from build123d import *

# Parameters (mm, degrees)
SKETCH1_W           = 565.88
SKETCH1_H           = 129.88
BOSS_EXTRUDE1_DEPTH = 3.5
SKETCH2_R           = 20
BOSS_EXTRUDE2_DEPTH = 14


with BuildPart() as part:
    # Sketch1 → Boss-Extrude1 (new, symmetric)
    with BuildSketch(Plane.XY):
        Rectangle(SKETCH1_W, SKETCH1_H)
    extrude(amount=BOSS_EXTRUDE1_DEPTH, both=True)

    # Sketch2 → Boss-Extrude2 (add)
    with BuildSketch(Plane.XY.offset(3.5)):
        with Locations((-70, 0)):
            Circle(SKETCH2_R)
    extrude(amount=BOSS_EXTRUDE2_DEPTH)


solid = part.part
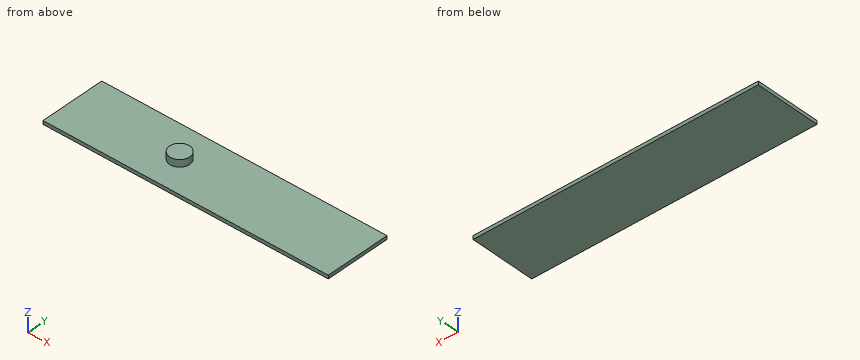
Can you work these out from the model? Positions are in its coordinate system, mm. Round coordinates to 2 decimals unless told otherwise and drop trailing zeros. Loops run counter-clockwise (first coordinate to the right, second up) from the corner with the lowest first, then second, coordinate; pieces in that order, holes last. Notation, with made-up numbers: (60.5, -30.5) - (111.5, -30.5) arc R12 cw to (111.5, -22.5) - close; hole circle Ø8 at (74.25, 26). An arc over 180 degrees is marked (long way). Answer in a Markdown table with one row per item. Add a question column.
Q1. I want a section at B-B on x = -70. List the corners of the cut face in (y, z) for me, and give its area (3 significant figures).
Q2. I want a section at D-D on y = -30. List the corners of the cut face in (x, z) for me, and give its area (3 significant figures).
Q3. I want a section at A-A on y = 0. List the corners of the cut face in (x, z) for me, and give its area (3 significant figures).
Q4. I need wall thicknesses on L1, parallel to Z at x = 21, y = -26.5; L2, parallel to X at y = 11, z = 7; L3, parallel to X at y = -13, z = 11.75. Which ranges of each line are inside material? Lowest first, please.
Q5. For pin 1 Ø10 at (x, y) = (153.5, -41) entering from +Z; pin 2 Ø6 at (y, z) = (-45.5, 4.5) entering from +X; pin 3 Ø1.5 at (y, z) = (42, 5) entering from -X, each with a flat end and sliding along its axis, tell me the tip position at first contact or that it passes through.
Q6. I want a section at C-C on z = 10.5. List the corners of the cut face in (x, y) for me, and give its area (3 significant figures).
A:
| question | item | result |
|---|---|---|
| 1 | outline | (-64.94, -3.5) - (64.94, -3.5) - (64.94, 3.5) - (20, 3.5) - (20, 17.5) - (-20, 17.5) - (-20, 3.5) - (-64.94, 3.5) - close |
| 1 | area | 1,470 mm^2 |
| 2 | outline | (-282.94, -3.5) - (282.94, -3.5) - (282.94, 3.5) - (-282.94, 3.5) - close |
| 2 | area | 3,960 mm^2 |
| 3 | outline | (-282.94, -3.5) - (282.94, -3.5) - (282.94, 3.5) - (-50, 3.5) - (-50, 17.5) - (-90, 17.5) - (-90, 3.5) - (-282.94, 3.5) - close |
| 3 | area | 4,520 mm^2 |
| 4 | L1 | -3.5 to 3.5 |
| 4 | L2 | -86.7 to -53.3 |
| 4 | L3 | -85.2 to -54.8 |
| 5 | pin 1 | z = 3.5 |
| 5 | pin 2 | x = 282.94 |
| 5 | pin 3 | through |
| 6 | outline | circle Ø40 at (-70, 0) |
| 6 | area | 1,260 mm^2 |
